For this review, use the dimensioned drawing (mm, ordinates from the lowest corner) and the shaded views. A direction names the side the tool comes from. Round coordinates to 2 decimals unless told otherwise and drop trailing zeros. Loops run counter-clockwise (first coordinate to the right, second up) from the corner with the lowest first, then second, coordinate; pieces in that order, holes last. Notation, with made-up numbers: (72.25, 12) - (90.25, 12) arc R31 ccw to (90.25, 40) - close; hole circle Ø2 at (11.5, 89.5). An arc over 180 degrees is marked (long way). Answer as CSV lines item,"result". Start each with the question number.
(1) Consider section A-A (z = 3). Give the boundary of the cut face in (x, y).
(2) Consider section B-B (x = 3). Give the boundary of the cut face in (y, z).
(3) Wall thickness on L1, parallel to Z at x = 1.6, y = 3.5; L2, parallel to Y at x = 1.15, z = 4.7; L3, parallel to X at y = 3.5, z = 2.05: over which ranges is each line inside the solid? List them lowest first.
(4) Consider section C-C (y = 7.25). Give the boundary of the cut face in (x, z), and give its area (3 significant figures).
(5) For the marked faces 1 and 2, list the 3-axis set-ups (+Z, -Z, +X, -X, +Y, -Y) from which the entire face can be reached by the end or side of a thin tool; tool diameter is ignored.
(6) Consider section D-D (y = 4.5). Give the boundary of the cut face in (x, z).
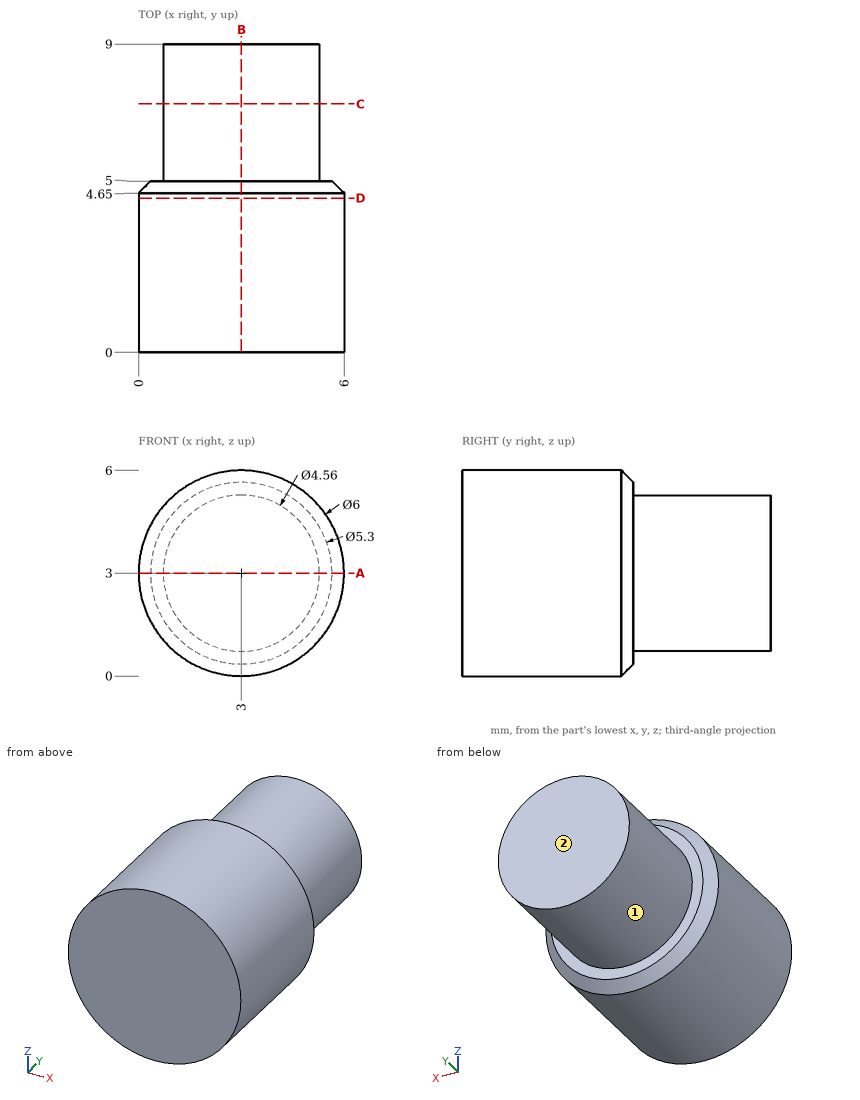
Determined:
1,outline,"(0, 0) - (6, 0) - (6, 4.65) - (5.65, 5) - (5.28, 5) - (5.28, 9) - (0.72, 9) - (0.72, 5) - (0.35, 5) - (0, 4.65) - close"
2,outline,"(0, 0) - (4.65, 0) - (5, 0.35) - (5, 0.72) - (9, 0.72) - (9, 5.28) - (5, 5.28) - (5, 5.65) - (4.65, 6) - (0, 6) - close"
3,L1,"z = 0.35 to 5.65"
3,L2,"y = 0 to 5"
3,L3,"x = 0.15 to 5.85"
4,outline,"circle Ø4.56 at (3, 3)"
4,area,"16.3 mm^2"
5,face 1,"+Y"
5,face 2,"+Z, -Z, +X, -X, +Y"
6,outline,"circle Ø6 at (3, 3)"
